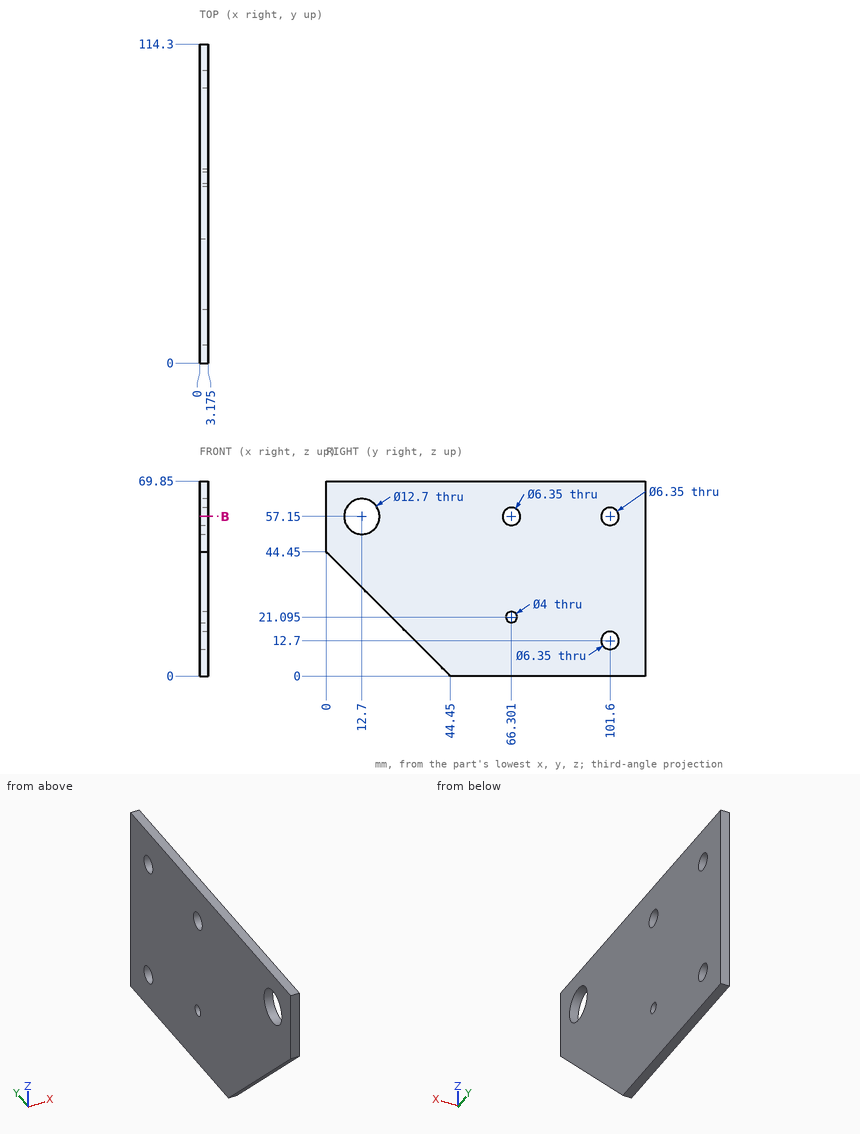
Design review of the part shown in the three views and the two pictorial views. Dimensions are in mm from the part's minimum x, y and z. Round coordinates to 2 decimals unless told otherwise and drop trailing zeros. Use a Markdown table: item, result. Add a question column.
Q1. We need section B-B, the plane z = 57.15. Count the separate pieces of the cut face and the enclosed holes in it, plus the area to 3 significant figures.
Q2. To check wall thickness, follow line 1 (Z direction, x = 2.8, y = 8); line 2 (Z direction, x = 1.4, y = 64); line 3 (Y direction, x = 2.9, z = 29.5). State the ranges of each line that lie inside material, in increasing order.
Q3. Insertion check: pin 1 (2.5 mm diameter, centred on y = 66.3, z = 21.09, fed in from -X); pin 2 (1 mm diameter, centred on x = 2, y = 33, fed in from -Z); pin 3 (1.5 mm diameter, centred on x = 2.5, y = 18.5, fed in from -Z). Each pin has a flat end and moves straight along its axis. Give the tip position at first contact, or say it passes through.
Findings below:
| question | item | result |
|---|---|---|
| 1 | separate pieces | 4 |
| 1 | enclosed holes | 0 |
| 1 | area | 282 mm² |
| 2 | line 1 | z = 36.45 to 52.88, 61.42 to 69.85 |
| 2 | line 2 | z = 0 to 54.96, 59.34 to 69.85 |
| 2 | line 3 | y = 14.95 to 114.3 |
| 3 | pin 1 | passes through |
| 3 | pin 2 | stops at z = 10.95 |
| 3 | pin 3 | stops at z = 25.2 |
